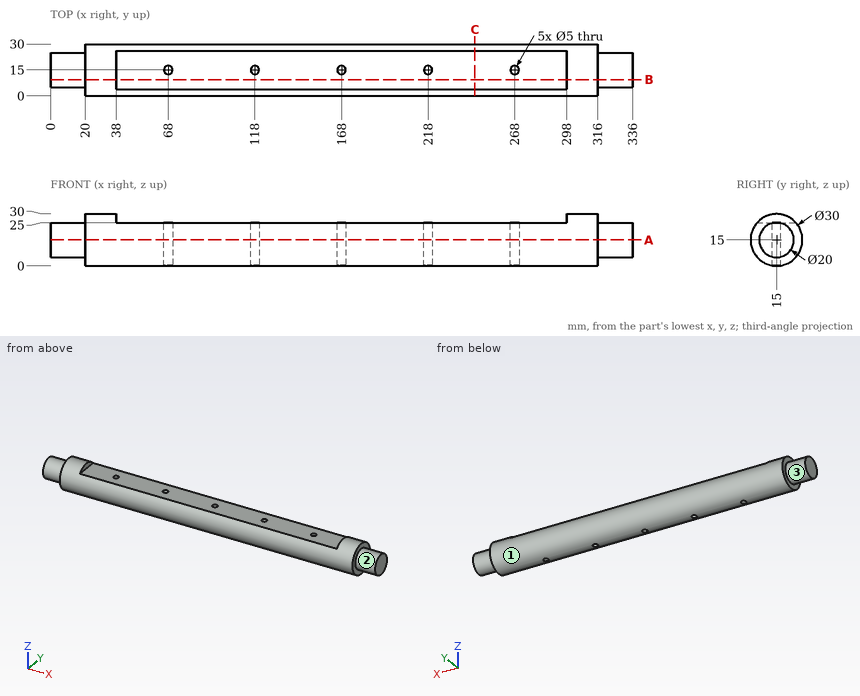
The drawing under review shows one solid part. Ordinate dimensions are in mm from its lowest x, y, z. A direction names the side the tool comes from. Coordinates: 2 decimals unless noted, no trailing zeros. Loops run counter-clockwise (first coordinate to the right, second up) from the corner with the lowest first, then second, coordinate; pieces in that order, holes last.
Item 1: Add section A-A (z = 15). Write out the cut boundary in (x, y), and give its area (3 significant figures).
Completed:
outline: (0, 5) - (20, 5) - (20, 0) - (316, 0) - (316, 5) - (336, 5) - (336, 25) - (316, 25) - (316, 30) - (20, 30) - (20, 25) - (0, 25) - close; hole circle Ø5 at (68, 15); hole circle Ø5 at (118, 15); hole circle Ø5 at (168, 15); hole circle Ø5 at (218, 15); hole circle Ø5 at (268, 15)
area: 9,580 mm2
Item 2: For the marked faces 1, 2 and 3, list the 3-axis set-ups (+Z, -Z, +X, -X, +Y, -Y) from which the entire face can be reached by the end or side of a thin tool; tool diameter is ignored.
Completed:
face 1: +X, -X
face 2: +X
face 3: -X
Item 3: Add section B-B (y = 9.5). Write out the cut boundary in (x, z).
Completed:
outline: (0, 6.65) - (20, 6.65) - (20, 1.04) - (316, 1.04) - (316, 6.65) - (336, 6.65) - (336, 23.35) - (316, 23.35) - (316, 28.96) - (298, 28.96) - (298, 25) - (38, 25) - (38, 28.96) - (20, 28.96) - (20, 23.35) - (0, 23.35) - close
Item 4: Wall thickness on L1, parallel to X at y = 28.5, z = 16.5; L2, parallel to Y at x = 68, z = 6.5; L3, parallel to Z at x = 55.5, y = 15.5: over which ranges is each line inside the solid? List them lowest first.
Completed:
L1: x = 20 to 316
L2: y = 2.64 to 12.5, 17.5 to 27.36
L3: z = 0.01 to 25
Item 5: Add section C-C (x = 245). Write out the cut boundary in (y, z), and give its area (3 significant figures).
Completed:
outline: (3.82, 25) arc R15 ccw (long way) to (26.18, 25) - close
area: 629 mm2
Item 6: Clearance check with flat-ended pins moving along their axes: pin 1 (4.5 mm diameter, centred on x = 118, y = 15, fed in from -Z); pin 2 (6.5 mm diameter, centred on x = 226.5, y = 9.5, fed in from +Z); pin 3 (1.5 mm diameter, centred on y = 12.5, z = 27.5, fed in from +X); pin 4 (2 mm diameter, centred on x = 87.5, z = 18, fed in from +Y). State where each tip first meets the part, or that it passes through.
Completed:
pin 1: passes through
pin 2: stops at z = 25
pin 3: stops at x = 316
pin 4: stops at y = 29.87
